from build123d import *

# Parameters (mm, degrees)
SKETCH1_W                    = 120
SKETCH1_H                    = 120
BOSS_EXTRUDE1_DEPTH          = 5
CSK_FOR_M6_SFHCS1_AT_2_COUNT = 2
CSK_FOR_M6_SFHCS1_AT_2_PITCH = 100
CSK_FOR_M6_SFHCS1_AT_3_COUNT = 2
CSK_FOR_M6_SFHCS1_AT_3_PITCH = 141.421356237
CSK_FOR_M6_SFHCS1_AT_4_COUNT = 2
CSK_FOR_M6_SFHCS1_AT_4_PITCH = 100
SKETCH5_W                    = 96
SKETCH5_H                    = 30
BOSS_EXTRUDE2_DEPTH          = 20
SKETCH6_R                    = 20
BOSS_EXTRUDE3_DEPTH          = 15
SKETCH7_R                    = 25
CUT_EXTRUDE2_DEPTH           = 7.5
SKETCH8_R                    = 8
CUT_EXTRUDE3_DEPTH           = 155.486245342
CHAMFER1_SIZE                = 1
CHAMFER1_SIZE_2              = 0.714285714
FILLET1_R                    = 15
CHAMFER2_SIZE                = 1


with BuildPart() as part:
    # Sketch1 → Boss-Extrude1 (new body)
    with BuildSketch(Plane.XY):
        Rectangle(SKETCH1_W, SKETCH1_H)
    extrude(amount=BOSS_EXTRUDE1_DEPTH)

    # Sketch4 → CSK for M6 SFHCS1 (revolve, cut)
    with BuildSketch(Plane(origin=(-50, 50, 5), x_dir=(0, -1, 0), z_dir=(1, 0, 0))):
        Polygon((0, 0), (0, 5), (3.3, 5), (3.3, 3.42), (6.72, 0), align=None)
    csk_for_m6_sfhcs1 = revolve(axis=Axis((-50, 50, 11.35), (0, 0, -1)), mode=Mode.SUBTRACT)

    # CSK for M6 SFHCS1 at 2: CSK for M6 SFHCS1 ×2
    with Locations(*[(i * CSK_FOR_M6_SFHCS1_AT_2_PITCH, 0, 0) for i in range(1, CSK_FOR_M6_SFHCS1_AT_2_COUNT)]):
        add(csk_for_m6_sfhcs1, mode=Mode.SUBTRACT)

    # CSK for M6 SFHCS1 at 3: CSK for M6 SFHCS1 ×2
    with Locations(*[Vector(0.7071067811865476, -0.7071067811865476, 0) * (i * CSK_FOR_M6_SFHCS1_AT_3_PITCH) for i in range(1, CSK_FOR_M6_SFHCS1_AT_3_COUNT)]):
        add(csk_for_m6_sfhcs1, mode=Mode.SUBTRACT)

    # CSK for M6 SFHCS1 at 4: CSK for M6 SFHCS1 ×2
    with Locations(*[(0, -i * CSK_FOR_M6_SFHCS1_AT_4_PITCH, 0) for i in range(1, CSK_FOR_M6_SFHCS1_AT_4_COUNT)]):
        add(csk_for_m6_sfhcs1, mode=Mode.SUBTRACT)

    # Sketch5 → Boss-Extrude2 (add, symmetric)
    with BuildSketch(Plane(origin=(0, 0, 0), x_dir=(0, 0, -1), z_dir=(1, 0, 0))):
        with Locations((-53, 0)):
            Rectangle(SKETCH5_W, SKETCH5_H)
    extrude(amount=BOSS_EXTRUDE2_DEPTH, both=True)

    # Sketch6 → Boss-Extrude3 (add, symmetric)
    with BuildSketch(Plane(origin=(0, 0, 0), x_dir=(1, 0, 0), z_dir=(0, 1, 0))):
        with Locations((0, -101)):
            Circle(SKETCH6_R)
    extrude(amount=BOSS_EXTRUDE3_DEPTH, both=True)

    # Sketch7 → Cut-Extrude2 (cut, symmetric)
    with BuildSketch(Plane(origin=(0, 0, 0), x_dir=(1, 0, 0), z_dir=(0, 1, 0))):
        with Locations((0, -101)):
            Circle(SKETCH7_R)
    extrude(amount=CUT_EXTRUDE2_DEPTH, both=True, mode=Mode.SUBTRACT)

    # Sketch8 → Cut-Extrude3 (cut, through all)
    with BuildSketch(Plane(origin=(0, 15, 0), x_dir=(1, 0, 0), z_dir=(0, 1, 0))):
        with Locations(Location((0, -101, 0), (0, 0, 270))):
            Circle(SKETCH8_R)
    extrude(amount=-CUT_EXTRUDE3_DEPTH, mode=Mode.SUBTRACT)

    # Chamfer1
    # the kernel refuses this chamfer: 1, 0.714285714 mm, written as the material it takes off along each edge
    with BuildSketch(Plane(origin=(-20, 15, 5), x_dir=(0, -1, 0), z_dir=(0, 0, 1))) as chamfer1_piece_1:
        Polygon((CHAMFER1_SIZE, 0), (0, CHAMFER1_SIZE), (0, 0), align=None)
    extrude(amount=96, mode=Mode.SUBTRACT)
    with BuildSketch(Plane(origin=(-20, -15, 101), x_dir=(1, 0, 0), z_dir=(0, 0, -1)), Plane(origin=(20, 15, 5), x_dir=(0, -1, 0), z_dir=(0, 0, 1)), Plane(origin=(20, -15, 101), x_dir=(0, 1, 0), z_dir=(0, 0, -1))) as chamfer1_piece_2:
        Polygon((CHAMFER1_SIZE, 0), (0, -CHAMFER1_SIZE), (0, 0), align=None)
    extrude(amount=96, mode=Mode.SUBTRACT)
    with BuildSketch(Plane(origin=(0, -15, 101), x_dir=(-1, 0, 0), z_dir=(0, 0, -1))) as chamfer1_piece_3:
        Polygon((20 - CHAMFER1_SIZE, 0), (20, CHAMFER1_SIZE), (20, 0), align=None)
    revolve(axis=Axis((0, -15, 101), (0, 1, 0)), revolution_arc=180, mode=Mode.SUBTRACT)
    with BuildSketch(Plane(origin=(0, 15, 101), x_dir=(-1, 0, 0), z_dir=(0, 0, -1))) as chamfer1_piece_4:
        Polygon((20 - CHAMFER1_SIZE, 0), (20, -CHAMFER1_SIZE), (20, 0), align=None)
    revolve(axis=Axis((0, 15, 101), (0, 1, 0)), revolution_arc=180, mode=Mode.SUBTRACT)
    with BuildSketch(Plane(origin=(0, 7.5, 101), x_dir=(-1, 0, 0), z_dir=(0, 0, -1))) as chamfer1_piece_5:
        Polygon((20 - CHAMFER1_SIZE, 0), (20, CHAMFER1_SIZE), (20, 0), align=None)
    revolve(axis=Axis((0, 7.5, 101), (0, 1, 0)), revolution_arc=180, mode=Mode.SUBTRACT)
    with BuildSketch(Plane(origin=(0, -7.5, 101), x_dir=(-1, 0, 0), z_dir=(0, 0, -1))) as chamfer1_piece_6:
        Polygon((20, -CHAMFER1_SIZE), (20 - CHAMFER1_SIZE, 0), (20, 0), align=None)
    revolve(axis=Axis((0, -7.5, 101), (0, 1, 0)), revolution_arc=180, mode=Mode.SUBTRACT)
    with BuildSketch(Plane(origin=(-20, -7.5, 83.428317012), x_dir=(0, -1, 0), z_dir=(0, 0, 1))) as chamfer1_piece_7_section:
        Polygon((CHAMFER1_SIZE, 0), (0, CHAMFER1_SIZE), (0, 0), align=None)
    chamfer1_piece_7 = extrude(amount=17.571682988, mode=Mode.PRIVATE)
    chamfer1_piece_7 = chamfer1_piece_7 & Plane(origin=(0, -7.5, 101), x_dir=(1, 0, 0), z_dir=(0, 1, 0)) * Cylinder(25, 40, mode=Mode.PRIVATE)
    add(chamfer1_piece_7, mode=Mode.SUBTRACT)
    with BuildSketch(Plane(origin=(20, 7.5, 83.428317012), x_dir=(0, 1, 0), z_dir=(0, 0, 1))) as chamfer1_piece_8_section:
        Polygon((CHAMFER1_SIZE, 0), (0, CHAMFER1_SIZE), (0, 0), align=None)
    chamfer1_piece_8 = extrude(amount=17.571682988, mode=Mode.PRIVATE)
    chamfer1_piece_8 = chamfer1_piece_8 & Plane(origin=(0, 7.5, 101), x_dir=(1, 0, 0), z_dir=(0, 1, 0)) * Cylinder(25, 40, mode=Mode.PRIVATE)
    add(chamfer1_piece_8, mode=Mode.SUBTRACT)
    with BuildSketch(Plane(origin=(20, -7.5, 83.428317012), x_dir=(0, -1, 0), z_dir=(0, 0, 1))) as chamfer1_piece_9_section:
        Polygon((CHAMFER1_SIZE, 0), (0, -CHAMFER1_SIZE), (0, 0), align=None)
    chamfer1_piece_9 = extrude(amount=17.571682988, mode=Mode.PRIVATE)
    chamfer1_piece_9 = chamfer1_piece_9 & Plane(origin=(0, -7.5, 101), x_dir=(1, 0, 0), z_dir=(0, 1, 0)) * Cylinder(25, 40, mode=Mode.PRIVATE)
    add(chamfer1_piece_9, mode=Mode.SUBTRACT)
    with BuildSketch(Plane(origin=(-20, 7.5, 83.428317012), x_dir=(0, 1, 0), z_dir=(0, 0, 1))) as chamfer1_piece_10_section:
        Polygon((CHAMFER1_SIZE, 0), (0, -CHAMFER1_SIZE), (0, 0), align=None)
    chamfer1_piece_10 = extrude(amount=17.571682988, mode=Mode.PRIVATE)
    chamfer1_piece_10 = chamfer1_piece_10 & Plane(origin=(0, 7.5, 101), x_dir=(1, 0, 0), z_dir=(0, 1, 0)) * Cylinder(25, 40, mode=Mode.PRIVATE)
    add(chamfer1_piece_10, mode=Mode.SUBTRACT)
    with BuildSketch(Plane(origin=(0, -15, 101), x_dir=(0, 0, 1), z_dir=(-1, 0, 0))) as chamfer1_piece_11:
        Polygon((8 + CHAMFER1_SIZE, 0), (8, CHAMFER1_SIZE), (8, 0), align=None)
    revolve(axis=Axis((0, -15, 101), (0, 1, 0)), mode=Mode.SUBTRACT)
    with BuildSketch(Plane(origin=(0, 15, 101), x_dir=(0, 0, 1), z_dir=(-1, 0, 0))) as chamfer1_piece_12:
        Polygon((8 + CHAMFER1_SIZE, 0), (8, -CHAMFER1_SIZE), (8, 0), align=None)
    revolve(axis=Axis((0, 15, 101), (0, 1, 0)), mode=Mode.SUBTRACT)
    with BuildSketch(Plane(origin=(-20, -7.5, 86), x_dir=(0, 0, -1), z_dir=(0, 1, 0))) as chamfer1_piece_13:
        with BuildLine():
            Line((CHAMFER1_SIZE, 0), (0.56416807, -0.43583193))
            ThreePointArc((0.56416807, -0.43583193), (0.281621078, -0.214347187), (0, 0))
            Line((0, 0), (CHAMFER1_SIZE, 0))
        make_face()
    extrude(amount=15, mode=Mode.SUBTRACT)
    with BuildSketch(Plane(origin=(20, -7.5, 86), x_dir=(0, 0, -1), z_dir=(0, 1, 0))) as chamfer1_piece_14:
        with BuildLine():
            Line((CHAMFER1_SIZE_2, 0), (0.80417029, 0.629192029))
            ThreePointArc((0.80417029, 0.629192029), (0.416667008, 0.319390803), (0, 0))
            Line((0, 0), (CHAMFER1_SIZE_2, 0))
        make_face()
    extrude(amount=15, mode=Mode.SUBTRACT)
    with BuildSketch(Plane(origin=(-20, -7.5, 83.428317012), x_dir=(0, -1, 0), z_dir=(0, 0, 1))) as chamfer1_piece_15a_section:
        Polygon((CHAMFER1_SIZE, 0), (0, CHAMFER1_SIZE), (0, 0), align=None)
    chamfer1_piece_15a = extrude(amount=17.571682988, mode=Mode.PRIVATE)
    chamfer1_piece_15a = chamfer1_piece_15a - Plane(origin=(0, -7.5, 101), x_dir=(1, 0, 0), z_dir=(0, 1, 0)) * Cylinder(25, 40, mode=Mode.PRIVATE)
    with BuildSketch(Plane(origin=(-20, -10.071682988, 86), x_dir=(0, 0, -1), z_dir=(0, 1, 0))) as chamfer1_piece_15b_section:
        with BuildLine():
            Line((CHAMFER1_SIZE, 0), (0.56416807, -0.43583193))
            ThreePointArc((0.56416807, -0.43583193), (0.281621078, -0.214347187), (0, 0))
            Line((0, 0), (CHAMFER1_SIZE, 0))
        make_face()
    chamfer1_piece_15b = extrude(amount=17.571682988, mode=Mode.PRIVATE)
    chamfer1_piece_15b = split(chamfer1_piece_15b, bisect_by=Plane(origin=(-20, -7.5, 86), z_dir=(0, -1, 0)), keep=Keep.TOP, mode=Mode.PRIVATE)
    chamfer1_piece_15 = chamfer1_piece_15a & chamfer1_piece_15b
    add(chamfer1_piece_15, mode=Mode.SUBTRACT)
    with BuildSketch(Plane(origin=(20, -7.5, 86), x_dir=(0, 0, -1), z_dir=(0, 1, 0))) as chamfer1_piece_16a_section:
        with BuildLine():
            Line((CHAMFER1_SIZE_2, 0), (0.80417029, 0.629192029))
            ThreePointArc((0.80417029, 0.629192029), (0.416667008, 0.319390803), (0, 0))
            Line((0, 0), (CHAMFER1_SIZE_2, 0))
        make_face()
    chamfer1_piece_16a = extrude(amount=17.625714283, mode=Mode.PRIVATE)
    chamfer1_piece_16a = split(chamfer1_piece_16a, bisect_by=Plane(origin=(20, 7.5, 86), z_dir=(0, 1, 0)), keep=Keep.TOP, mode=Mode.PRIVATE)
    with BuildSketch(Plane(origin=(20, 7.5, 83.428317012), x_dir=(0, 1, 0), z_dir=(0, 0, 1))) as chamfer1_piece_16b_section:
        Polygon((CHAMFER1_SIZE, 0), (0, CHAMFER1_SIZE), (0, 0), align=None)
    chamfer1_piece_16b = extrude(amount=17.571682988, mode=Mode.PRIVATE)
    chamfer1_piece_16b = chamfer1_piece_16b - Plane(origin=(0, 7.5, 101), x_dir=(1, 0, 0), z_dir=(0, 1, 0)) * Cylinder(25, 40, mode=Mode.PRIVATE)
    chamfer1_piece_16 = chamfer1_piece_16a & chamfer1_piece_16b
    add(chamfer1_piece_16, mode=Mode.SUBTRACT)
    with BuildSketch(Plane(origin=(20, -7.5, 83.428317012), x_dir=(0, -1, 0), z_dir=(0, 0, 1))) as chamfer1_piece_17a_section:
        Polygon((CHAMFER1_SIZE, 0), (0, -CHAMFER1_SIZE), (0, 0), align=None)
    chamfer1_piece_17a = extrude(amount=17.571682988, mode=Mode.PRIVATE)
    chamfer1_piece_17a = chamfer1_piece_17a - Plane(origin=(0, -7.5, 101), x_dir=(1, 0, 0), z_dir=(0, 1, 0)) * Cylinder(25, 40, mode=Mode.PRIVATE)
    with BuildSketch(Plane(origin=(20, -10.125714283, 86), x_dir=(0, 0, -1), z_dir=(0, 1, 0))) as chamfer1_piece_17b_section:
        with BuildLine():
            Line((CHAMFER1_SIZE_2, 0), (0.80417029, 0.629192029))
            ThreePointArc((0.80417029, 0.629192029), (0.416667008, 0.319390803), (0, 0))
            Line((0, 0), (CHAMFER1_SIZE_2, 0))
        make_face()
    chamfer1_piece_17b = extrude(amount=17.625714283, mode=Mode.PRIVATE)
    chamfer1_piece_17b = split(chamfer1_piece_17b, bisect_by=Plane(origin=(20, -7.5, 86), z_dir=(0, -1, 0)), keep=Keep.TOP, mode=Mode.PRIVATE)
    chamfer1_piece_17 = chamfer1_piece_17a & chamfer1_piece_17b
    add(chamfer1_piece_17, mode=Mode.SUBTRACT)
    with BuildSketch(Plane(origin=(-20, -7.5, 86), x_dir=(0, 0, -1), z_dir=(0, 1, 0))) as chamfer1_piece_18a_section:
        with BuildLine():
            Line((CHAMFER1_SIZE, 0), (0.56416807, -0.43583193))
            ThreePointArc((0.56416807, -0.43583193), (0.281621078, -0.214347187), (0, 0))
            Line((0, 0), (CHAMFER1_SIZE, 0))
        make_face()
    chamfer1_piece_18a = extrude(amount=17.571682988, mode=Mode.PRIVATE)
    chamfer1_piece_18a = split(chamfer1_piece_18a, bisect_by=Plane(origin=(-20, 7.5, 86), z_dir=(0, 1, 0)), keep=Keep.TOP, mode=Mode.PRIVATE)
    with BuildSketch(Plane(origin=(-20, 7.5, 83.428317012), x_dir=(0, 1, 0), z_dir=(0, 0, 1))) as chamfer1_piece_18b_section:
        Polygon((CHAMFER1_SIZE, 0), (0, -CHAMFER1_SIZE), (0, 0), align=None)
    chamfer1_piece_18b = extrude(amount=17.571682988, mode=Mode.PRIVATE)
    chamfer1_piece_18b = chamfer1_piece_18b - Plane(origin=(0, 7.5, 101), x_dir=(1, 0, 0), z_dir=(0, 1, 0)) * Cylinder(25, 40, mode=Mode.PRIVATE)
    chamfer1_piece_18 = chamfer1_piece_18a & chamfer1_piece_18b
    add(chamfer1_piece_18, mode=Mode.SUBTRACT)

    # Fillet1
    fillet1_edges = [part.edges().sort_by_distance(p)[0] for p in [
        (-19.5, -14.5, 5),
        (19.5, -14.5, 5),
        (-19.5, 14.5, 5),
        (19.5, 14.5, 5),
        (20, 0, 5),
        (-20, 0, 5),
        (0, 15, 5),
        (0, -15, 5),
    ]]
    fillet(fillet1_edges, radius=FILLET1_R)

    # Chamfer2
    chamfer2_edges = [part.edges().sort_by_distance(p)[0] for p in [
        (60, 0, 5),
        (0, 60, 5),
        (-60, 0, 5),
        (0, -60, 5),
    ]]
    chamfer(chamfer2_edges, length=CHAMFER2_SIZE)


solid = part.part
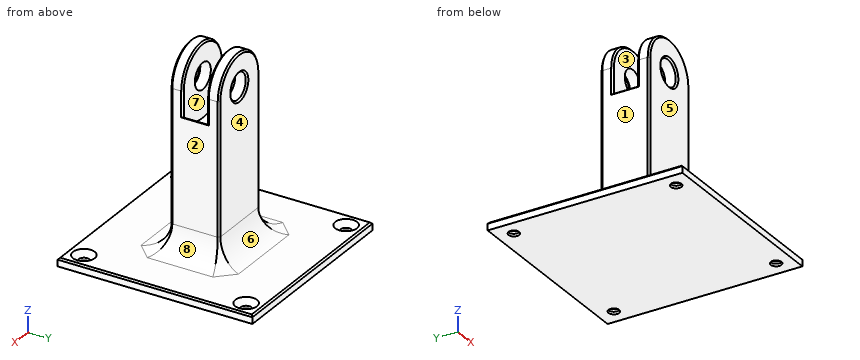
Verification items for the finished model (mm, model axes). Face numbers are marked on the shaded views. A direction names the side the tool comes from. Give positions to 0.01 mm unless a question says otherwise; leave off trailing zeros. Write each loop counter-clockwise with the first axis right and the second up, starting at its lowest first coordinate (ties: lowest second). Pieces come first, ordered by that corner, then holes.
(1) Cross-section at B-B (y = 50). Enter the section's corners in (x, z).
(2) Cross-section at C-C (z = 50.5). Enter the section's corners in (x, y), plus the area to 3 significant figures.
(3) Access from +Z, -Z, +X, -X, +Y, -Y to the whole of each face (thin tool, end or side, straight path). Record for the marked faces 1, 2, 3, 4 and 5.
(4) Mould release check, pull along Y, two halves, no side actions. Record for the marked faces 6, 7 and 8: +Y half, -Y half, draft (parallel to the pull), parting line (faces both ways), or undercut.
(5) Material ranges on line 1 (X direction, y = -50, z = 1); line 2 (Y direction, x = -12, z = 105.5), recorded low to high.
(6) Gauge pin test, flat ends, axial feed: pin 1 (2 mm diameter, centred on x = -31, y = -29, fed in from -Z); pin 2 (1 mm diameter, centred on x = -11.5, z = 51.5, fed in from +Y); pin 3 (10 mm diameter, centred on x = 24, z = 15.5, fed in from -Y); pin 4 (14 mm diameter, centred on y = 6.5, z = 46.5, fed in from -X). Record the tip position at first contact, or that the pin passes through.
(7) Cross-section at A-A (x = 0). State how many separate pieces and enclosed holes the cut face has, plus the area to 3 significant figures.
(8) Cross-section at D-D (y = 5.5). Enter the section's corners in (x, z).
Worked out:
1. outline: (-60, 0) - (-53.3, 0) - (-53.3, 1.58) - (-56.72, 5) - (-59, 5) - (-60, 4) - close; (-46.7, 0) - (46.7, 0) - (46.7, 1.58) - (43.28, 5) - (-43.28, 5) - (-46.7, 1.58) - close; (53.3, 0) - (60, 0) - (60, 4) - (59, 5) - (56.72, 5) - (53.3, 1.58) - close
2. outline: (-20, -14) - (-19, -15) - (19, -15) - (20, -14) - (20, 14) - (19, 15) - (-19, 15) - (-20, 14) - close
2. area: 1,200 mm2
3. face 1: +Z, -X, +Y, -Y
3. face 2: +Z, +X, +Y, -Y
3. face 3: +Z
3. face 4: +Z, +X, -X, +Y
3. face 5: +Z, +X, -X, -Y
4. face 6: +Y half
4. face 7: undercut
4. face 8: draft
5. line 1: x = -60 to -53.3, -46.7 to 46.7, 53.3 to 60
5. line 2: y = -15 to -7.5, 7.5 to 15
6. pin 1: stops at z = 0
6. pin 2: stops at y = 15
6. pin 3: stops at y = -16.85
6. pin 4: stops at x = -20
7. separate pieces: 3
7. enclosed holes: 0
7. area: 3,260 mm2
8. outline: (-60, 0) - (60, 0) - (60, 4) - (59, 5) - (35, 5) arc R15 cw to (20, 20) - (20, 85.29) - (19.37, 85.2) arc R25 cw to (-19.56, 85.44) - (-20, 85) - (-20, 20) arc R15 cw to (-35, 5) - (-59, 5) - (-60, 4) - close
